Source: CAD feature listing. Evaluate the final solid. Frame: model axes, mm. Face numbers are marked on the shaded views. A direction names the side the tool comes from. Give positions to 0.01 mm unless a question says otherwise; leave off trailing zeros. Write each loop counter-clockwise with the first axis right and the second up, starting at its lowest first coordinate (ties: lowest second). Pieces come first, ordered by that corner, then holes. Notation, with made-up numbers: M 40.5,25.5 L 78.5,25.5 A33 cw 78.5,53.5 Z; hole C 34,8.25 d2. An arc over 180 degrees is marked long. Return JSON: item names as keys, results as strings.
Autodesk Inventor part; units mm, degrees
ref_plane "YZ Plane" through (0, 0, 0) normal (1, 0, 0) x (0, 1, 0)
ref_plane "XZ Plane" through (0, 0, 0) normal (0, 1, 0) x (-1, 0, 0)
ref_plane "XY Plane" through (0, 0, 0) normal (0, 0, 1) x (1, 0, 0)
sketch "Skizze1" plane through (0, 0, 0) normal (0, 0, 1) x (1, 0, 0)
  circle A0 centre (0, 0) radius 15
  circle A1 centre (0, 0) radius 4
  line L0 (0, 0) -> (15, 0) construction
  line L1 (-9.6418, 11.4907) -> (66.0959, 75.0422) construction
  line L2 (-9.6418, -11.4907) -> (66.0959, -75.0422) construction
  line L3 (66.0959, 75.0422) -> (66.0959, -75.0422) construction
  arc A2 (66.0959, -75.0422) -> (66.0959, 75.0422) centre (0, 0) ccw
  arc A3 (46.6507, -58.7257) -> (46.6507, 58.7257) centre (0, 0) ccw
  line L4 (46.6507, 58.7257) -> (66.0959, 75.0422)
  line L5 (46.6507, -58.7257) -> (66.0959, -75.0422)
  arc A4 (51.0992, 29.2211) -> (57.1349, 48.586) centre (47.9933, 40.8122) ccw
  line L6 (-3.8823, 14.4889) -> (51.0992, 29.2211)
  line L7 (-3.8823, -14.4889) -> (51.0992, -29.2211)
  arc A5 (57.1349, -48.586) -> (51.0992, -29.2211) centre (47.9933, -40.8122) ccw
  line L8 (30, 0) -> (60, 0) construction
  line L9 (30, 3.5) -> (60, 3.5)
  line L10 (60, -3.5) -> (30, -3.5)
  arc A6 (30, 3.5) -> (30, -3.5) centre (30, 0) ccw
  arc A7 (60, -3.5) -> (60, 3.5) centre (60, 0) ccw
  line L11 (0, 0) -> (66.0959, 0) construction
  arc A8 (56.3733, -66.8839) -> (56.3733, 66.8839) centre (0, 0) ccw construction
  circle A9 centre (67.9788, 55.0481) radius 4
  line L12 (67.9788, 55.0481) -> (0, 0) construction
  circle A10 centre (80.2782, 34.7395) radius 4
  circle A11 centre (86.6631, 11.8714) radius 4
  circle A12 centre (86.6631, -11.8714) radius 4
  circle A13 centre (80.2782, -34.7395) radius 4
  circle A14 centre (67.9788, -55.0481) radius 4
  line L13 (2.6458, 3) -> (-2.6458, 3)
  point P0 (75, 0)
  point P1 (45, 0)
  dimension "d0" = 8
  dimension "d1" = 30
  dimension "d2" = 40
  dimension "d3" = 100
  dimension "d4" = 25
  dimension "d5" = 12
  dimension "d6" = 15
  dimension "d7" = 12
  dimension "d8" = 15
  dimension "d10" = 60
  dimension "d13" = 0
  dimension "d14" = 30
  dimension "d15" = 7
  dimension "d16" = 30
  dimension "d27" = 8
  dimension "d28" = 80
  dimension "d29" = 1
  dimension "d32" = 78
  dimension "d35" = 3
extrude "Extrusion1" add sketch "Skizze1" along normal blind 10 contours A0 | A0 L6 A4 A3 A5 L7 | A3 L4 A2 L5 | L13 A1 picked at (-0.6179, 3.1815)
fillet "Rundung1" radius 4 4 edges at (66.0959, 75.0422, 5) (66.0959, -75.0422, 5) (46.6507, 58.7257, 5) (46.6507, -58.7257, 5)
equation "\"d7\" = d5"
equation "\"d8\" = d6"
properties part number "ParallelMecha_Capstondisc_V3"
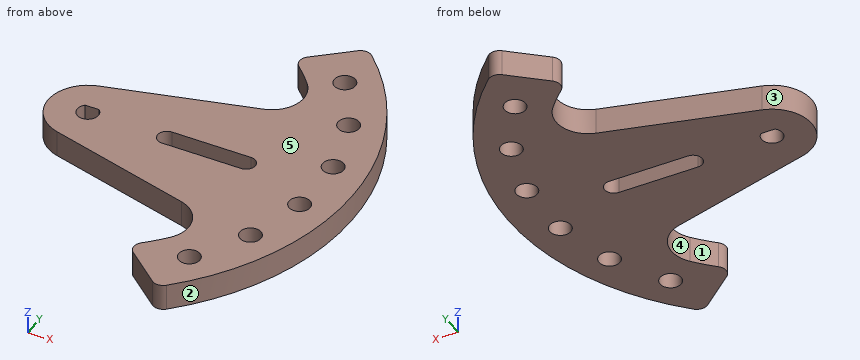
1) Contact query for flat-ended pins moving along their axis: pin 1 Ø3 at (x, z) = (62.5, 7) entering from -Y; pin 2 Ø2 at (y, z) = (46.5, 6.5) entering from +X; pin 3 Ø5 at (y, z) = (-41, 5.5) entering from -X. Output: stop coordinate, or through.
Numbers:
{"pin 1": "stops at y = -73.2", "pin 2": "stops at x = 89.05", "pin 3": "stops at x = 59.69"}
2) Set-up query: the marked faces 1 and 2. Return all of +Z, -Z, +X, -X, +Y, -Y with unobstructed straight access to the full face (end or side cutting, diameter ignored); none if empty.
Numbers:
{"face 1": "+Z, -Z, -X", "face 2": "+Z, -Z, +X"}
3) Draft query along Y for the marked faces 3, 4 and 5. Return one class per face: released by +Y, released by -Y, zero draft, split by the parting line, or undercut.
Numbers:
{"face 3": "split by the parting line", "face 4": "undercut", "face 5": "zero draft"}
4) Line query: line 1 (Y direction, x = 57, z = 1.75); line 2 (Y direction, x = 53, z = 1.75); line 3 (Y direction, x = 47.5, z = 7.25). Output: solid intervals per line, ascending. Write a range as [from, to].
Numbers:
{"line 1": "y = [-67.41, -48.74], [-32.88, -3.5], [3.5, 32.88], [48.74, 67.41]", "line 2": "y = [-64.05, -53.07], [-29.91, -3.5], [3.5, 29.91], [53.07, 64.05]", "line 3": "y = [-28.26, -3.5], [3.5, 28.26]"}
5) Cut plane D-D, the plane x = 35. Return the cut outline in (y, z), then the cut area to 3 significant figures.
Numbers:
{"outline": "M -24.91,0 L -3.5,0 L -3.5,10 L -24.91,10 Z; M 3.5,0 L 24.91,0 L 24.91,10 L 3.5,10 Z", "area": "428 mm²"}
6) Cut plane A-A, the plane y = 0. Return the cut outline in (x, z).
Numbers:
{"outline": "M -15,0 L -4,0 L -4,10 L -15,10 Z; M 4,0 L 26.5,0 L 26.5,10 L 4,10 Z; M 63.5,0 L 100,0 L 100,10 L 63.5,10 Z"}
7) Cut plane B-B, the plane x = 0. Return the cut outline in (y, z), then the cut area to 3 significant figures.
Numbers:
{"outline": "M -15.53,0 L -4,0 L -4,10 L -15.53,10 Z; M 3,0 L 15.53,0 L 15.53,10 L 3,10 Z", "area": "241 mm²"}
8) Cut plane C-C, the plane z = 7.25. Give the number of separate pieces and of enclosed holes in the cut face, then the cut area to 3 significant figures.
Numbers:
{"separate pieces": "1", "enclosed holes": "8", "area": "7,340 mm²"}
